Part model, mm, in its own coordinate system. A direction names the side the tool comes from. Coordinates: 2 decimals unless noted, no trailing zeros. Write each loop counter-clockwise with the first axis right and the second up, starting at its lowest first coordinate (ties: lowest second). Pieces come first, ordered by that corner, then holes. Notation, with made-up numbers: M -37.5,19 L 6.5,19 A17 ccw 6.5,38 Z; hole C -18.75,69.5 d8. An arc over 180 degrees is marked long. Use a Markdown table: item, result. Add a question column.
Q1. Slice it at B-B on x = 9. Write the cut outline in (y, z).
Q2. Slice it at A-A on y = -6.5. Write the cut outline in (x, z), then the cut area to 3 significant figures.
Q3. Slice it at C-C on z = 62.5. Write the cut outline in (x, y).
Q4. Slice it at D-D on x = -38.5. Write the cut outline in (y, z), then the cut area to 3 significant figures.
Q5. Pin check, flat tips, straight feed: pin 1 Ø5 at (x, z) = (9, 175) entering from -Y; pin 2 Ø13 at (x, z) = (-9, 175) entering from -Y; pin 3 Ø11.5 at (x, z) = (0, 86.45) entering from +Y; pin 4 Ø1.6 at (y, z) = (-1, 48.5) entering from -X. Stop position of each tip, or through.
Q6. Wall check: L1, parallel to X at y = -6.25, z = 58; L2, parallel to Z at x = -17, y = -0.75; L3, parallel to Y at x = -22.5, z = 70.5. Give the ranges that are in metal, low to high. Write a range as from..to.
Q7. Mould opens along Z. For faces 1 (the flat face through (50, -6, 99)), 2 (the cylindrical face through (21.93, -0.74, 136.85)), 3 (the flat face through (0, -1, 200)) say: released by +Z, released by -Z, zero draft, split by the parting line, or undercut.
Q8. Tool access for faces 4 (the cylindrical face through (43.35, -0.74, 2.97)), 5 (the flat face through (48.5, -7, 99)): list every direction of +Z, -Z, +X, -X, +Y, -Y with a clear straight run to the whole face (end or side of a thin tool).
from build123d import *

# Parameters (mm, degrees)
EXTRUDE_1_DEPTH     = 200
SKETCH_2_R          = 1.7
CUT_EXTRUDE_1_DEPTH = 10
FILLET_1_R          = 2
SKETCH_5_R          = 1.7
SKETCH_5_R_2        = 1.2
SKETCH_5_R_3        = 4
CUT_EXTRUDE_2_DEPTH = 10
SKETCH_7_R          = 1.1
SKETCH_7_R_2        = 2.1
CUT_EXTRUDE_3_DEPTH = 10
SKETCH_11_R         = 5
SKETCH_11_R_2       = 1.65
CUT_EXTRUDE_4_DEPTH = 10
SKETCH_12_R         = 1.6
CUT_EXTRUDE_5_DEPTH = 10


with BuildPart() as part:
    # Эскиз1 → Вытянуть1 (new body)
    with BuildSketch(Plane.XY):
        with BuildLine():
            Line((-47, 0), (47, 0))
            ThreePointArc((47, 0), (49.121320344, -0.878679656), (50, -3))
            Line((50, -3), (50, -10))
            Line((50, -10), (48.5, -10))
            Line((48.5, -10), (48.5, -3))
            ThreePointArc((48.5, -3), (48.060660172, -1.939339828), (47, -1.5))
            Line((47, -1.5), (-47, -1.5))
            ThreePointArc((-47, -1.5), (-48.060660172, -1.939339828), (-48.5, -3))
            Line((-48.5, -3), (-48.5, -10))
            Line((-48.5, -10), (-50, -10))
            Line((-50, -10), (-50, -3))
            ThreePointArc((-50, -3), (-49.121320344, -0.878679656), (-47, 0))
        make_face()
    extrude(amount=EXTRUDE_1_DEPTH)

    # Эскиз2 → Вырез-Вытянуть1 (cut)
    with BuildSketch(Plane(origin=(0, 0, 0), x_dir=(1, 0, 0), z_dir=(0, 1, 0))):
        with Locations(Location((-42, -4, 0), (0, 0, 180))):
            Circle(SKETCH_2_R)
        with Locations(Location((42, -4, 0), (0, 0, 180))):
            Circle(SKETCH_2_R)
        with Locations(Location((42, -196, 0), (0, 0, 270))):
            Circle(SKETCH_2_R)
        with Locations(Location((-42, -196, 0), (0, 0, 270))):
            Circle(SKETCH_2_R)
    extrude(amount=-CUT_EXTRUDE_1_DEPTH, mode=Mode.SUBTRACT)

    # Скругление1
    fillet_1_edges = [part.edges().sort_by_distance(p)[0] for p in [
        (-49.25, -10, 200),
        (49.25, -10, 0),
        (-49.25, -10, 0),
        (49.25, -10, 200),
    ]]
    fillet(fillet_1_edges, radius=FILLET_1_R)

    # Эскиз5 → Вырез-Вытянуть2 (cut)
    with BuildSketch(Plane(origin=(0, 0, 0), x_dir=(-1, 0, 0), z_dir=(0, 1, 0))):
        with Locations((-23.5, 137.5)):
            Circle(SKETCH_5_R)
        with Locations((23.5, 137.5)):
            Circle(SKETCH_5_R)
        with Locations((-22, 170)):
            Circle(SKETCH_5_R_2)
        with Locations((22, 170)):
            Circle(SKETCH_5_R_2)
        with Locations((-9, 175)):
            Circle(SKETCH_5_R_3)
        with Locations((9, 175)):
            Circle(SKETCH_5_R_3)
        with BuildLine():
            Line((-20.35129058, 133.635803619), (-19.624017853, 141.635803619))
            ThreePointArc((-19.624017853, 141.635803619), (-19.141685475, 142.607633836), (-18.130178043, 143))
            Line((-18.130178043, 143), (18.130178043, 143))
            ThreePointArc((18.130178043, 143), (19.141685475, 142.607633836), (19.624017853, 141.635803619))
            Line((19.624017853, 141.635803619), (20.35129058, 133.635803619))
            ThreePointArc((20.35129058, 133.635803619), (19.965084606, 132.488492568), (18.85745077, 132))
            Line((18.85745077, 132), (-18.85745077, 132))
            ThreePointArc((-18.85745077, 132), (-19.965084606, 132.488492568), (-20.35129058, 133.635803619))
        make_face()
    extrude(amount=-CUT_EXTRUDE_2_DEPTH, mode=Mode.SUBTRACT)

    # Эскиз7 → Вырез-Вытянуть3 (cut)
    with BuildSketch(Plane(origin=(0, 0, 0), x_dir=(-1, 0, 0), z_dir=(0, 1, 0))):
        with Locations(Location((20, 50, 0), (0, 0, 90))):
            Circle(SKETCH_7_R)
        with Locations(Location((-20, 50, 0), (0, 0, 90))):
            Circle(SKETCH_7_R)
        with Locations((0, 7.5)):
            Circle(SKETCH_7_R_2)
        with BuildLine():
            Line((-11.5, 40), (11.5, 40))
            ThreePointArc((11.5, 40), (13.267766953, 40.732233047), (14, 42.5))
            Line((14, 42.5), (14, 57.5))
            ThreePointArc((14, 57.5), (13.267766953, 59.267766953), (11.5, 60))
            Line((11.5, 60), (-11.5, 60))
            ThreePointArc((-11.5, 60), (-13.267766953, 59.267766953), (-14, 57.5))
            Line((-14, 57.5), (-14, 42.5))
            ThreePointArc((-14, 42.5), (-13.267766953, 40.732233047), (-11.5, 40))
        make_face()
    extrude(amount=-CUT_EXTRUDE_3_DEPTH, mode=Mode.SUBTRACT)

    # Эскиз11 → Вырез-Вытянуть4 (cut)
    with BuildSketch(Plane(origin=(0, 0, 0), x_dir=(-1, 0, 0), z_dir=(0, 1, 0))):
        with Locations((0, 98.55)):
            Circle(SKETCH_11_R)
        with Locations((0, 86.45)):
            Circle(SKETCH_11_R)
        with Locations((0, 74.35)):
            Circle(SKETCH_11_R)
        with Locations((0, 110.65)):
            Circle(SKETCH_11_R)
        with Locations((10, 98.55)):
            Circle(SKETCH_11_R_2)
        with Locations((10, 74.35)):
            Circle(SKETCH_11_R_2)
        with Locations((10, 86.45)):
            Circle(SKETCH_11_R_2)
        with Locations(Location((10, 110.65, 0), (0, 0, 90))):
            Circle(SKETCH_11_R_2)
    extrude(amount=-CUT_EXTRUDE_4_DEPTH, mode=Mode.SUBTRACT)

    # Эскиз12 → Вырез-Вытянуть5 (cut)
    with BuildSketch(Plane.ZY.offset(50)):
        with Locations((100, -6.5)):
            Circle(SKETCH_12_R)
    extrude(amount=-CUT_EXTRUDE_5_DEPTH, mode=Mode.SUBTRACT)


solid = part.part
Recorded:
| question | item | result |
|---|---|---|
| 1 | outline | M -1.5,0 L 0,0 L 0,40 L -1.5,40 Z; M -1.5,60 L 0,60 L 0,132 L -1.5,132 Z; M -1.5,143 L 0,143 L 0,171 L -1.5,171 Z; M -1.5,179 L 0,179 L 0,200 L -1.5,200 Z |
| 2 | outline | M -50,0 L -48.5,0 L -48.5,98.4 L -50,98.4 Z; M -50,101.6 L -48.5,101.6 L -48.5,200 L -50,200 Z; M 48.5,0 L 50,0 L 50,200 L 48.5,200 Z |
| 2 | area | 595 mm² |
| 3 | outline | M -50,-10 L -48.5,-10 L -48.5,-3 A1.5 cw -47,-1.5 L 47,-1.5 A1.5 cw 48.5,-3 L 48.5,-10 L 50,-10 L 50,-3 A3 ccw 47,0 L -47,0 A3 ccw -50,-3 Z |
| 4 | outline | M -1.5,0 L 0,0 L 0,200 L -1.5,200 Z |
| 4 | area | 300 mm² |
| 5 | pin 1 | through |
| 5 | pin 2 | y = -1.5 |
| 5 | pin 3 | y = 0 |
| 5 | pin 4 | x = -49.75 |
| 6 | L1 | -50..-48.5, 48.5..50 |
| 6 | L2 | 0..132, 143..200 |
| 6 | L3 | -1.5..0 |
| 7 | face 1 | zero draft |
| 7 | face 2 | undercut |
| 7 | face 3 | released by +Z |
| 8 | face 4 | +Y, -Y |
| 8 | face 5 | +Z, -Z, -Y |
